```python
from build123d import *

# Parameters (mm, degrees)
SKETCH1_R           = 2
BOSS_EXTRUDE1_DEPTH = 6
SKETCH2_W           = 20
SKETCH2_H           = 6
BOSS_EXTRUDE2_DEPTH = 20
SKETCH3_R           = 6.25
CUT_EXTRUDE1_DEPTH  = 6
FILLET1_R           = 3
FILLET2_R           = 3
FILLET3_R           = 3


with BuildPart() as part:
    # Sketch1 → Boss-Extrude1 (new body)
    with BuildSketch(Plane.XY):
        with BuildLine():
            Line((-20, 70), (20, 70))
            Line((20, 70), (20, 55))
            Line((20, 55), (15, 55))
            ThreePointArc((15, 55), (11.464466094, 53.535533906), (10, 50))
            Line((10, 50), (10, 32))
            Line((10, 32), (-10, 32))
            Line((-10, 32), (-10, 50))
            ThreePointArc((-10, 50), (-11.464466094, 53.535533906), (-15, 55))
            Line((-15, 55), (-20, 55))
            Line((-20, 55), (-20, 70))
        make_face()
        with Locations((-8, 62.5)):
            Circle(SKETCH1_R, mode=Mode.SUBTRACT)
        with Locations((8, 62.5)):
            Circle(SKETCH1_R, mode=Mode.SUBTRACT)
    extrude(amount=BOSS_EXTRUDE1_DEPTH)

    # Sketch2 → Boss-Extrude2 (add)
    with BuildSketch(Plane(origin=(0, 0, 0), x_dir=(-1, 0, 0), z_dir=(0, 0, -1))):
        with Locations((0, 35)):
            Rectangle(SKETCH2_W, SKETCH2_H)
    extrude(amount=BOSS_EXTRUDE2_DEPTH)

    # Sketch3 → Cut-Extrude1 (cut)
    with BuildSketch(Plane(origin=(0, 38, 0), x_dir=(1, 0, 0), z_dir=(0, 1, 0))):
        with Locations((0, 9.85)):
            Circle(SKETCH3_R)
    extrude(amount=-CUT_EXTRUDE1_DEPTH, mode=Mode.SUBTRACT)

    # Fillet1
    fillet1_edges = [part.edges().sort_by_distance(p)[0] for p in [
        (10, 35, -20),
        (-10, 35, -20),
    ]]
    fillet(fillet1_edges, radius=FILLET1_R)

    # Fillet2
    fillet2_edges = [part.edges().sort_by_distance(p)[0] for p in [
        (0, 38, 0),
    ]]
    fillet(fillet2_edges, radius=FILLET2_R)

    # Fillet3
    fillet3_edges = [part.edges().sort_by_distance(p)[0] for p in [
        (0, 32, 6),
    ]]
    fillet(fillet3_edges, radius=FILLET3_R)


solid = part.part
```
Here's how the part is built. I have some questions about the finished solid (model axes, mm). A direction names the side the tool comes from. Give positions to 0.01 mm unless a question says otherwise; leave off trailing zeros. Loops run counter-clockwise (first coordinate to the right, second up) from the corner with the lowest first, then second, coordinate; pieces in that order, holes last. Notation, with made-up numbers: M 36.5,-22.75 L 48.5,-22.75 A15 ccw 48.5,1.25 Z; hole C -17,17 d9. An arc over 180 degrees is marked long. Use one line per item in the form item = value. Start each with the question number.
Q1. Thinking about a two-plate mould opening in Y: for faces 5 (the cylindrical face through (-8.26, 64.483, 2.958)), 6 (the flat face through (-20, 62, 3)), 7 (the cylindrical face through (-0.14, 32.86, 5.1)), 8 (the flat face through (0, 70, 3)), which applies, +Y half, -Y half, draft (parallel to the pull), parting line (faces both ways), or undercut?
Q2. If we section it at B-B (x = 0): Write out the boundary of the cut face in (y, z).
Q3. If we section it at C-C (y = 62): Write out the boundary of the cut face in (x, z).
Q4. I need wall thicknesses on line 1 along Z through (x, y) = (0, 36.55); line 2 along Y through (x, z) = (-8, 2.1); line 3 along X through (y, z) = (36.2, -9.85). Which ranges of each line are inside material? Lowest first, please.
Q5. Which directions (+Z, -Z, +X, -X, +Y, -Y) give clear straight access to the entire face, cutting with the end or side of a thin tool? Please do faces 1 (the flat face through (0, 59, 0)), 2 (the flat face through (0, 32, -3)), 3 (the flat face through (10, 37, -3)), 4 (the flat face through (-17, 55, 3)).
Q6. Will these pins go through, and if not, where does the flat tip stop? pin 1 Ø1 at (x, z) = (-2.5, -3) entering from +Y; pin 2 Ø12 at (y, z) = (40, -16) entering from -X; pin 3 Ø1.5 at (x, z) = (-17.5, 1.5) entering from -Y.
Q7. If we section it at A-A (z = 1.75): Write out the boundary of the cut face in (x, y).
Q8. If we section it at D-D (z = -9.85): Write out the boundary of the cut face in (x, y), then the cut area to 3 significant figures.
Taken from the geometry:
q1.face_5 = undercut
q1.face_6 = draft
q1.face_7 = -Y half
q1.face_8 = +Y half
q2.outline = M 32,-20 L 38,-20 L 38,-16.1 L 32,-16.1 Z; M 32,-3.6 L 38,-3.6 L 38,-3 A3 cw 41,0 L 70,0 L 70,6 L 35,6 A3 ccw 32,3 Z
q3.outline = M -20,0 L -9.94,0 L -9.94,6 L -20,6 Z; M -6.06,0 L 6.06,0 L 6.06,6 L -6.06,6 Z; M 9.94,0 L 20,0 L 20,6 L 9.94,6 Z
q4.line_1 = -20 to -16.1, -3.6 to 6
q4.line_2 = 32 to 60.5, 64.5 to 70
q4.line_3 = -10 to -6.25, 6.25 to 10
q5.face_1 = -Z, +X, -X, +Y
q5.face_2 = +Z, -Z, +X, -X, -Y
q5.face_3 = +Z, -Z, +X, -Y
q5.face_4 = +Z, -Z, -X, -Y
q6.pin_1 = 38.04
q6.pin_2 = -10
q6.pin_3 = 55
q7.outline = M -20,55 L -15,55 A5 cw -10,50 L -10,32 L 10,32 L 10,50 A5 cw 15,55 L 20,55 L 20,70 L -20,70 Z; hole C -8,62.5 d4; hole C 8,62.5 d4
q8.outline = M -10,32 L -6.25,32 L -6.25,38 L -10,38 Z; M 6.25,32 L 10,32 L 10,38 L 6.25,38 Z
q8.area = 45.0 mm^2
